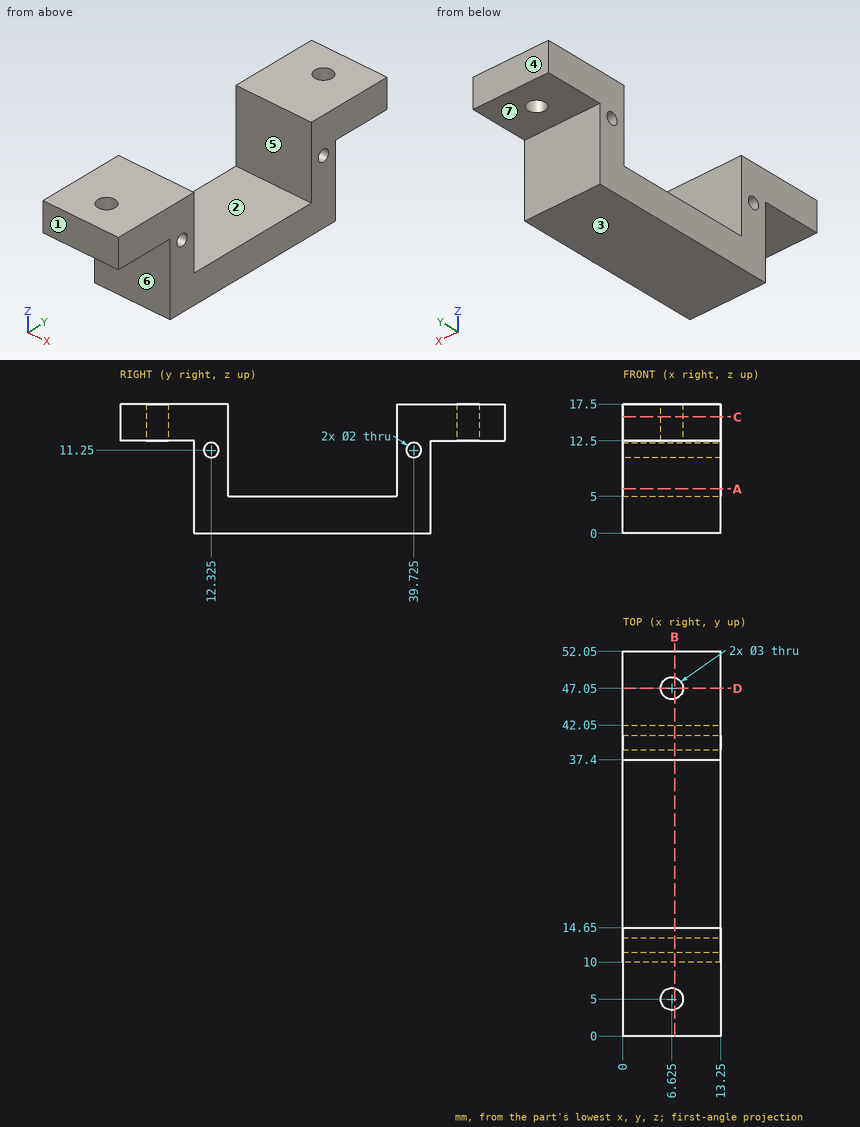
Source: three-view drawing plus pictorial views. Frame: mm from the lowest corner of the part. A direction names the side the tool comes from. Coordinates: 2 decimals unless noted, no trailing zeros. Order: outer loops, then holes, each group sorted by start corner. A loop starts at its lowest first (then second) coordinate and runs counter-clockwise, first axis right, second up.
Item 1: Set-up query: the marked faces 5, 6 and 7. Return all of +Z, -Z, +X, -X, +Y, -Y with unobstructed straight access to the full face (end or side cutting, diameter ignored); none if empty.
Output values:
face 5: +Z, +X, -X
face 6: -Z, +X, -X, -Y
face 7: -Z, +X, -X, +Y
Item 2: Material intervals for line 1 (Y direction, x = 4, z = 11.25) (3 decimals); line 2 (Y direction, x = 9.5, z = 13); line 3 (Z direction, x = 11, y = 30), sorted ascending.
Output values:
line 1: y = 10 to 11.325, 13.325 to 14.65, 37.4 to 38.725, 40.725 to 42.05
line 2: y = 0 to 14.65, 37.4 to 52.05
line 3: z = 0 to 5
Item 3: Cut plane A-A (z = 6). Return loops of the section in (x, y).
Output values:
outline: (0, 10) - (13.25, 10) - (13.25, 14.65) - (0, 14.65) - close; (0, 37.4) - (13.25, 37.4) - (13.25, 42.05) - (0, 42.05) - close
Item 4: Cut plane B-B (x = 7). Return loops of the section in (y, z) (3 decimals).
Output values:
outline: (0, 12.5) - (3.548, 12.5) - (3.548, 17.5) - (0, 17.5) - close; (6.452, 12.5) - (10, 12.5) - (10, 0) - (42.05, 0) - (42.05, 12.5) - (45.598, 12.5) - (45.598, 17.5) - (37.4, 17.5) - (37.4, 5) - (14.65, 5) - (14.65, 17.5) - (6.452, 17.5) - close; (48.502, 12.5) - (52.05, 12.5) - (52.05, 17.5) - (48.502, 17.5) - close; hole circle Ø2 at (12.325, 11.25); hole circle Ø2 at (39.725, 11.25)
Item 5: Cut plane C-C (z = 15.75). Return loops of the section in (x, y) (3 decimals).
Output values:
outline: (0, 0) - (13.25, 0) - (13.25, 14.65) - (0, 14.65) - close; (0, 37.4) - (13.25, 37.4) - (13.25, 52.05) - (0, 52.05) - close; hole circle Ø3 at (6.625, 5); hole circle Ø3 at (6.625, 47.05)
Item 6: First-contact query: P1, Ø4, axis at x = 7, z = 5.5, coming from the -Y side; P2, Ø6, axis at y = 30, z = 9.5, coming from the +X side; P3, Ø3, axis at x = 3.5, y = 5.5, coming from the -Z side; P4, Ø6.5, axis at x = 8, y = 26.5, coming from the +Z side. Flat tips, straight axial feed; report the tip coordinate or a pass-through.
Output values:
P1: stops at y = 10
P2: passes through
P3: stops at z = 12.5
P4: stops at z = 5
Item 7: Pull-direction query (Y, two-part tool) for the marked faces 1, 2, 3 and 4; classes: pulls with the +Y half, pulls with the -Y half, needs draft (parallel to the pull), parting line crosses it, or undercut.
Output values:
face 1: pulls with the -Y half
face 2: undercut
face 3: needs draft
face 4: pulls with the +Y half
Item 8: Cut plane D-D (y = 47.05). Return loops of the section in (x, z) (3 decimals).
Output values:
outline: (0, 12.5) - (5.125, 12.5) - (5.125, 17.5) - (0, 17.5) - close; (8.125, 12.5) - (13.25, 12.5) - (13.25, 17.5) - (8.125, 17.5) - close
